The model under review builds one solid part; all positions refer to its coordinate system, in mm. Give positions to 0.01 mm unless a question says otherwise; leave off trailing zeros. Order: outer loops, then holes, each group sorted by start corner. A loop starts at its lowest first (then second) coordinate and runs counter-clockwise, first axis right, second up. Notation, with made-up numbers: (66.5, 60.5) - (93.5, 60.5) arc R11 cw to (93.5, 68.5) - close; hole circle Ø11 at (29.25, 42.25). An arc over 180 degrees is marked (long way). Use a Markdown table: item, result. Add a question column.
```python
from build123d import *

# Parameters (mm, degrees)
SKETCH4_R           = 2
BOSS_EXTRUDE3_DEPTH = 6
SKETCH6_R           = 3.276903459
BOSS_EXTRUDE4_DEPTH = 6
CUT_EXTRUDE2_DEPTH  = 10


with BuildPart() as part:
    # Sketch4 → Boss-Extrude3 (new body)
    with BuildSketch(Plane.XY):
        with BuildLine():
            ThreePointArc((11.330682707, 3.9516616), (8.917819898, 4.428819506), (6.681915604, 3.403968986))
            ThreePointArc((6.681915604, 3.403968986), (6.066818441, 4.407801607), (5.302192362, 5.302995112))
            ThreePointArc((5.302192362, 5.302995112), (6.967815552, 7.112770233), (7.259627029, 9.554989032))
            ThreePointArc((7.259627029, 9.554989032), (7.053423028, 9.708203932), (6.843986457, 9.856969584))
            ThreePointArc((6.843986457, 9.856969584), (4.61147306, 8.824753264), (3.40498051, 6.681400208))
            ThreePointArc((3.40498051, 6.681400208), (2.317318441, 7.131972816), (1.172541409, 7.406763642))
            ThreePointArc((1.172541409, 7.406763642), (1.456299749, 9.849931218), (0.256880001, 11.997250213))
            ThreePointArc((0.256880001, 11.997250213), (0, 12), (-0.256880001, 11.997250213))
            ThreePointArc((-0.256880001, 11.997250213), (-1.456299749, 9.849931218), (-1.172541409, 7.406763642))
            ThreePointArc((-1.172541409, 7.406763642), (-2.317318441, 7.131972816), (-3.404980509, 6.681400207))
            ThreePointArc((-3.404980509, 6.681400207), (-4.61147306, 8.824753264), (-6.843986457, 9.856969584))
            ThreePointArc((-6.843986457, 9.856969584), (-7.053423028, 9.708203933), (-7.259627029, 9.554989032))
            ThreePointArc((-7.259627029, 9.554989032), (-6.967815552, 7.112770233), (-5.302192362, 5.302995112))
            ThreePointArc((-5.302192362, 5.302995112), (-6.066818441, 4.407801607), (-6.681915604, 3.403968986))
            ThreePointArc((-6.681915604, 3.403968986), (-8.917819898, 4.428819506), (-11.330682707, 3.9516616))
            ThreePointArc((-11.330682707, 3.9516616), (-11.412678196, 3.708203933), (-11.489443278, 3.463046803))
            ThreePointArc((-11.489443278, 3.463046803), (-9.817862641, 1.658772773), (-7.406586048, 1.173662691))
            ThreePointArc((-7.406586048, 1.173662691), (-7.499, 0), (-7.406586048, -1.173662691))
            ThreePointArc((-7.406586048, -1.173662691), (-9.817862641, -1.658772773), (-11.489443278, -3.463046803))
            ThreePointArc((-11.489443278, -3.463046803), (-11.412678196, -3.708203933), (-11.330682707, -3.9516616))
            ThreePointArc((-11.330682707, -3.9516616), (-8.917819898, -4.428819506), (-6.681915604, -3.403968986))
            ThreePointArc((-6.681915604, -3.403968986), (-6.066818441, -4.407801607), (-5.302192362, -5.302995112))
            ThreePointArc((-5.302192362, -5.302995112), (-6.967815552, -7.112770233), (-7.259627029, -9.554989032))
            ThreePointArc((-7.259627029, -9.554989032), (-7.053423028, -9.708203932), (-6.843986457, -9.856969584))
            ThreePointArc((-6.843986457, -9.856969584), (-4.61147306, -8.824753264), (-3.404980509, -6.681400207))
            ThreePointArc((-3.404980509, -6.681400207), (-2.317318441, -7.131972816), (-1.172541409, -7.406763642))
            ThreePointArc((-1.172541409, -7.406763642), (-1.456299749, -9.849931218), (-0.256880001, -11.997250213))
            ThreePointArc((-0.256880001, -11.997250213), (0, -12), (0.256880001, -11.997250213))
            ThreePointArc((0.256880001, -11.997250213), (1.456299749, -9.849931218), (1.172541409, -7.406763642))
            ThreePointArc((1.172541409, -7.406763642), (2.317318441, -7.131972816), (3.404980509, -6.681400207))
            ThreePointArc((3.404980509, -6.681400207), (4.61147306, -8.824753264), (6.843986457, -9.856969584))
            ThreePointArc((6.843986457, -9.856969584), (7.053423027, -9.708203933), (7.259627029, -9.554989032))
            ThreePointArc((7.259627029, -9.554989032), (6.967815552, -7.112770233), (5.302192362, -5.302995112))
            ThreePointArc((5.302192362, -5.302995112), (6.066818441, -4.407801607), (6.681915604, -3.403968986))
            ThreePointArc((6.681915604, -3.403968986), (8.917819898, -4.428819506), (11.330682707, -3.9516616))
            ThreePointArc((11.330682707, -3.9516616), (11.412678196, -3.708203932), (11.489443278, -3.463046803))
            ThreePointArc((11.489443278, -3.463046803), (9.817862641, -1.658772773), (7.406586048, -1.173662691))
            ThreePointArc((7.406586048, -1.173662691), (7.499, 0), (7.406586048, 1.173662691))
            ThreePointArc((7.406586048, 1.173662691), (9.817862641, 1.658772773), (11.489443278, 3.463046803))
            ThreePointArc((11.489443278, 3.463046803), (11.412678196, 3.708203932), (11.330682707, 3.9516616))
        make_face()
        Circle(SKETCH4_R, mode=Mode.SUBTRACT)
    extrude(amount=BOSS_EXTRUDE3_DEPTH)

    # Sketch6 → Boss-Extrude4 (add)
    with BuildSketch(Plane.XY.offset(6)):
        Circle(SKETCH6_R)
    extrude(amount=-BOSS_EXTRUDE4_DEPTH)

    # Sketch7 → Cut-Extrude2 (cut)
    with BuildSketch(Plane.XY.offset(6)):
        with BuildLine():
            Line((-1.710555465, 1.545), (1.710555465, 1.545))
            ThreePointArc((1.710555465, 1.545), (0, -2.305), (-1.710555465, 1.545))
        make_face()
    extrude(amount=-CUT_EXTRUDE2_DEPTH, mode=Mode.SUBTRACT)


solid = part.part
```
Q1. We need section C-C (y = 8.5). Write out the cut boundary in (x, z), plus the area to 3 significant figures.
Q2. Wall thickness on probe 1 along Y at (x, z) = (0, 4) (3 decimals); probe 2 along X at (y, z) = (0, 4.3) (3 decimals); probe 3 along X at (y, z) = (3.5, 3.8): over which ranges is each line inside the solid? List them lowest first.
Q3. We need section B-B (x = -2). Write out the cut boundary in (y, z).
Q4. We need section D-D (x = 4.25). Write out the cut boundary in (y, z), plus the area to 3 significant figures.
Q5. We need section A-A (y = 0). Write out the cut boundary in (x, z) (3 decimals).
Q6. Clearance check with flat-ended pins moving along their axes: P1, Ø3, axis at x = 7.5, z = 3, coming from the +Y side; P2, Ø3, axis at y = -5, z = 4.5, coming from the -X side; P3, Ø1.5, axis at x = 6, z = 2, coming from the -Y side. State where each tip first meets the part, or that it passes through.
Q7. Draft analysis for pull direction X (two halves, no side actions). For faces 1 (the flat face through (-3, 0, 6)), 2 (the cylindrical face through (6.08, 4.39, 2.96)), 3 (the cylindrical face through (2.333, 7.127, 2.958)), state which applies: pulls with the +X half, pulls with the -X half, needs draft (parallel to the pull), parting line crosses it, or undercut.
Here are the results:
| question | item | result |
|---|---|---|
| 1 | outline | (-7.32, 0) - (-4.3, 0) - (-4.3, 6) - (-7.32, 6) - close; (-1.49, 0) - (1.49, 0) - (1.49, 6) - (-1.49, 6) - close; (4.3, 0) - (7.32, 0) - (7.32, 6) - (4.3, 6) - close |
| 1 | area | 54.2 mm2 |
| 2 | probe 1 | -12 to -2.305, 1.545 to 12 |
| 2 | probe 2 | -7.499 to -2.305, 2.305 to 7.499 |
| 2 | probe 3 | -11.48 to -6.79, -6.63 to 6.63, 6.79 to 11.48 |
| 3 | outline | (-7.23, 0) - (-1.15, 0) - (-1.15, 6) - (-7.23, 6) - close; (1.15, 0) - (7.23, 0) - (7.23, 6) - (1.15, 6) - close |
| 4 | outline | (-8.44, 0) - (8.44, 0) - (8.44, 6) - (-8.44, 6) - close |
| 4 | area | 101 mm2 |
| 5 | outline | (-7.499, 0) - (-2.305, 0) - (-2.305, 6) - (-7.499, 6) - close; (2.305, 0) - (7.499, 0) - (7.499, 6) - (2.305, 6) - close |
| 6 | P1 | y = 9.86 |
| 6 | P2 | x = -11.48 |
| 6 | P3 | y = -9.84 |
| 7 | face 1 | needs draft |
| 7 | face 2 | undercut |
| 7 | face 3 | undercut |
